The model under review builds one solid part; all positions refer to its coordinate system, in mm. A direction names the side the tool comes from. Round coordinates to 2 decimals unless told otherwise and drop trailing zeros. Loops run counter-clockwise (first coordinate to the right, second up) from the corner with the lowest first, then second, coordinate; pieces in that order, holes last. Notation, with made-up numbers: M -37.75,-17 L 16.25,-17 A25 ccw 16.25,20 Z; hole C 12,51.5 d4. An arc over 180 degrees is marked long. Return JSON: item names as keys, results as strings. Group by question number.
Q1. Consider section C-C (z = 4.25). State the section outline as (x, y) points.
Q2. Draft analysis for pull direction X (two halves, no side actions). For faces 1 (the face through (13.163, -5.458, 3.296)), 2 (the face through (22.055, 1.551, 7.715)), 3 (the face through (-22.645, 1, 3)), state which applies: pulls with the +X half, pulls with the -X half, needs draft (parallel to the pull), parting line crosses it, or undercut.
Q3. For faces 4 (the face through (13, -7, 6.5)), 5 (the face through (13.455, -16.142, 4.056)), list the 3-axis set-ups (+Z, -Z, +X, -X, +Y, -Y) from which the entire face can be reached by the end or side of a thin tool; tool diameter is ignored.
Q4. Consider section B-B (x = 0). State the section outline as (y, z) points.
Q5. Clearance check with flat-ended pins moving along their axes: pin 1 Ø8 at (x, y) = (-13.5, 9) entering from -Z; pin 2 Ø10 at (x, y) = (7.5, -1.5) entering from +Z. State where each tip first meets the part, or that it passes through.
Q6. To check wall thickness, follow line 1 along Y through (x, z) = (15, 2.75); line 2 along Y through (x, z) = (16, 3.25); line 3 along X through (y, z) = (16.5, 4.5). State the ranges of each line that lie inside material, in increasing order.
Q7. Consider section A-A (y = 0). State the section outline as (x, z) points.
from build123d import *

# Parameters (mm, degrees)
F0_W          = 45
F0_H          = 45
F1_DEPTH      = 8
F2_R          = 14.25
F3_DEPTH      = 69
F3_DEPTH_BACK = 8
F4_W          = 45
F4_H          = 45
F4_R          = 15.5
F5_DEPTH      = 1.5
F6_R          = 1
F7_R          = 2
F8_DEPTH      = 8
F9_DEPTH      = 1.5


# Not quite as in the source:
# - an extrude ends at something that could not be found from the text; its depth is read off the source's solid


with BuildPart() as f1:
    # F0 (on Top) → F1 (new body)
    with BuildSketch(Plane.XY):
        with Locations((-0.144558493, 1.2362819078)):
            Rectangle(F0_W, F0_H)
    extrude(amount=F1_DEPTH)

    # F2 (on face) → F3 (cut, two sides)
    with BuildSketch(Plane.XY.offset(8)) as f3_sk:
        Circle(F2_R)
    extrude(amount=F3_DEPTH, mode=Mode.SUBTRACT)
    extrude(f3_sk.sketch, amount=-F3_DEPTH_BACK, mode=Mode.SUBTRACT)

    # F4 (on face) → F5 (cut)
    with BuildSketch(Plane.XY.offset(8)):
        with Locations((-0.144558493, 1.2362819078)):
            Rectangle(F4_W, F4_H)
        Circle(F4_R, mode=Mode.SUBTRACT)
    extrude(amount=F5_DEPTH, mode=Mode.SUBTRACT)

    # F6
    f6_edges = [f1.edges().sort_by_distance(p)[0] for p in [
        (-0.144558, 23.736282, 8),
        (-22.644558, 1.236282, 8),
        (-0.144558, -21.263718, 8),
        (22.355442, 1.236282, 8),
    ]]
    fillet(f6_edges, radius=F6_R)

    # F7 (on face) → F8 (cut)
    with BuildSketch(Plane.XY.offset(8)):
        with Locations((-15.1081832213, 15)):
            Circle(F7_R)
        with Locations((14.8917229997, 15.0750115548)):
            Circle(F7_R)
        with Locations((15.0417456403, -14.9246133297)):
            Circle(F7_R)
        with Locations((-15.1081832213, -15)):
            Circle(F7_R)
    extrude(amount=-F8_DEPTH, mode=Mode.SUBTRACT)

    # F4 (on face) → F9 (cut)
    with BuildSketch(Plane.XY.offset(8)):
        Circle(F4_R)
    extrude(amount=-F9_DEPTH, mode=Mode.SUBTRACT)


solid = f1.part
Values:
{
 "1": {"outline": "M -22.64,-21.26 L 22.36,-21.26 L 22.36,23.74 L -22.64,23.74 Z; hole C -15.11,-15 d4; hole C -15.11,15 d4; hole C 0,0 d28.5; hole C 14.89,15.08 d4; hole C 15.04,-14.92 d4"},
 "2": {"face 1": "undercut", "face 2": "pulls with the +X half", "face 3": "pulls with the -X half"},
 "3": {"face 4": "+Z", "face 5": "+Z, -Z"},
 "4": {"outline": "M -21.26,0 L -14.25,0 L -14.25,6.5 L -15.5,6.5 L -15.5,8 L -20.26,8 A1 ccw -21.26,7 Z; M 14.25,0 L 23.74,0 L 23.74,7 A1 ccw 22.74,8 L 15.5,8 L 15.5,6.5 L 14.25,6.5 Z"},
 "5": {"pin 1": "stops at z = 0", "pin 2": "passes through"},
 "6": {"line 1": "y = -21.26 to -16.92, -12.93 to 13.08, 17.07 to 23.74", "line 2": "y = -21.26 to -16.68, -13.17 to 13.41, 16.74 to 23.74", "line 3": "x = -22.64 to -16.43, -13.79 to 13.49, 16.3 to 22.36"},
 "7": {"outline": "M -22.64,0 L -14.25,0 L -14.25,6.5 L -15.5,6.5 L -15.5,8 L -21.64,8 A1 ccw -22.64,7 Z; M 14.25,0 L 22.36,0 L 22.36,7 A1 ccw 21.36,8 L 15.5,8 L 15.5,6.5 L 14.25,6.5 Z"}
}
